```python
from build123d import *

# Parameters (mm, degrees)
F0_R     = 3.175
F0_R_2   = 25.781
F1_DEPTH = 6.35


with BuildPart() as f1:
    # F0 (on Top) → F1 (new body)
    with BuildSketch(Plane.XY):
        with BuildLine():
            Line((139.7, 0), (12.7, 0))
            ThreePointArc((12.7, 0), (3.719744, -3.719744), (0, -12.7))
            Line((0, -12.7), (0, -139.7))
            ThreePointArc((0, -139.7), (3.719744, -148.680256), (12.7, -152.4))
            Line((12.7, -152.4), (139.7, -152.4))
            ThreePointArc((139.7, -152.4), (148.680256, -148.680256), (152.4, -139.7))
            Line((152.4, -139.7), (152.4, -12.7))
            ThreePointArc((152.4, -12.7), (148.680256, -3.719744), (139.7, 0))
        make_face()
        with Locations((12.7, -139.7)):
            Circle(F0_R, mode=Mode.SUBTRACT)
        with Locations((139.7, -139.7)):
            Circle(F0_R, mode=Mode.SUBTRACT)
        with Locations((76.2, -76.2)):
            Circle(F0_R_2, mode=Mode.SUBTRACT)
        with Locations((12.7, -12.7)):
            Circle(F0_R, mode=Mode.SUBTRACT)
        with Locations((139.7, -12.7)):
            Circle(F0_R, mode=Mode.SUBTRACT)
    extrude(amount=F1_DEPTH)


solid = f1.part
```
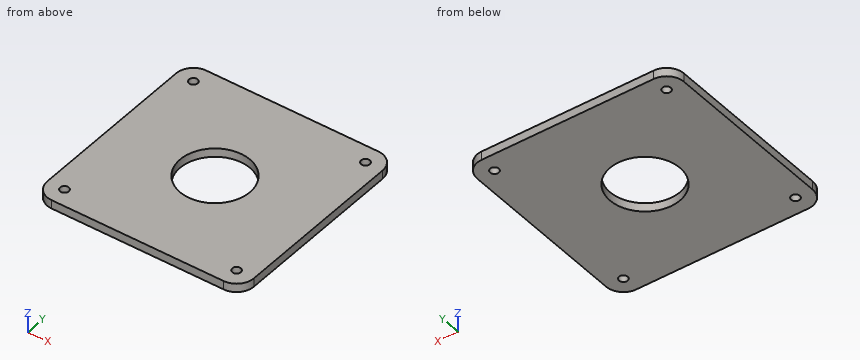
Verification items for the finished model (mm, model axes). Round coordinates to 2 decimals unless told otherwise and drop trailing zeros. Loops run counter-clockwise (first coordinate to the right, second up) from the corner with the lowest first, then second, coordinate; pieces in that order, holes last. Notation, with made-up numbers: (24.25, 89.25) -> (58.25, 89.25) arc R16 cw to (58.25, 108.25) -> close; hole circle Ø2 at (6.5, -33.75). An arc over 180 degrees is marked (long way). Answer as a JSON object with one key per item and string values.
Q1. Section check C-C (z = 1.5). Record the boundary of the cut face in (x, y) (3 decimals).
Data:
{"outline": "(0, -139.7) arc R12.7 ccw to (12.7, -152.4) -> (139.7, -152.4) arc R12.7 ccw to (152.4, -139.7) -> (152.4, -12.7) arc R12.7 ccw to (139.7, 0) -> (12.7, 0) arc R12.7 ccw to (0, -12.7) -> close; hole circle Ø6.35 at (12.7, -139.7); hole circle Ø6.35 at (12.7, -12.7); hole circle Ø51.562 at (76.2, -76.2); hole circle Ø6.35 at (139.7, -139.7); hole circle Ø6.35 at (139.7, -12.7)"}
Q2. Section check B-B (x = 76.2). Record the boundary of the cut face in (y, z), then the cut area to 3 significant figures.
Data:
{"outline": "(-152.4, 0) -> (-101.98, 0) -> (-101.98, 6.35) -> (-152.4, 6.35) -> close; (-50.42, 0) -> (0, 0) -> (0, 6.35) -> (-50.42, 6.35) -> close", "area": "640 mm2"}
Q3. Go/stop test with a flat-tipped pin: P1, Ø4, axis at x = 12.7, y = -139.7, coming from the +Z side. Record where the tip stops, or that it passes through.
Data:
{"P1": "passes through"}
Q4. Scan lines: line 1 (X direction, y = -139.7, z = 5) (3 decimals); line 2 (Y direction, x = 12.7, z = 2.5) (3 decimals); line 3 (X direction, y = -77.5, z = 1). Record each from-to range of solid material in increasing order. Write a range as from..to.
Data:
{"line 1": "x = 0..9.525, 15.875..136.525, 142.875..152.4", "line 2": "y = -152.4..-142.875, -136.525..-15.875, -9.525..0", "line 3": "x = 0..50.45, 101.95..152.4"}
Q5. Section check A-A (y = -76.2). Record the boundary of the cut face in (x, z), then the cut area to 3 significant figures.
Data:
{"outline": "(0, 0) -> (50.42, 0) -> (50.42, 6.35) -> (0, 6.35) -> close; (101.98, 0) -> (152.4, 0) -> (152.4, 6.35) -> (101.98, 6.35) -> close", "area": "640 mm2"}
